```python
from build123d import *

# Parameters (mm, degrees)
SKETCH7_R           = 4.826
BOSS_EXTRUDE2_DEPTH = 9.652
SKETCH11_R          = 3.937
BOSS_EXTRUDE3_DEPTH = 7.874
RIB1_REACH          = 117.25
SKETCH16_WALL_W     = 293.372991472
SKETCH16_WALL_H     = 7.874
SKETCH17_R          = 9.525
SKETCH17_R_2        = 6.35
BOSS_EXTRUDE4_DEPTH = 14.986
SKETCH18_R          = 9.525
SKETCH18_R_2        = 6.35
BOSS_EXTRUDE5_DEPTH = 14.986


with BuildPart() as part:
    # Sketch7 → Boss-Extrude2 (new body)
    with BuildSketch(Plane(origin=(0, 0, 0), x_dir=(1, 0, 0), z_dir=(0, 1, 0))):
        with BuildLine():
            Line((-34.925, 38.1), (34.925, 38.1))
            ThreePointArc((34.925, 38.1), (43.905256121, 34.380256121), (47.625, 25.4))
            Line((47.625, 25.4), (47.625, -25.4))
            ThreePointArc((47.625, -25.4), (43.905256121, -34.380256121), (34.925, -38.1))
            Line((34.925, -38.1), (-34.925, -38.1))
            ThreePointArc((-34.925, -38.1), (-43.905256121, -34.380256121), (-47.625, -25.4))
            Line((-47.625, -25.4), (-47.625, 25.4))
            ThreePointArc((-47.625, 25.4), (-43.905256121, 34.380256121), (-34.925, 38.1))
        make_face()
        with Locations(Location((-34.925, 25.4, 0), (0, 0, 270))):
            Circle(SKETCH7_R, mode=Mode.SUBTRACT)
        with Locations(Location((34.925, 25.4, 0), (0, 0, 90))):
            Circle(SKETCH7_R, mode=Mode.SUBTRACT)
        with Locations(Location((34.925, -25.4, 0), (0, 0, 270))):
            Circle(SKETCH7_R, mode=Mode.SUBTRACT)
        with Locations(Location((-34.925, -25.4, 0), (0, 0, 90))):
            Circle(SKETCH7_R, mode=Mode.SUBTRACT)
    extrude(amount=-BOSS_EXTRUDE2_DEPTH)



with BuildPart() as body_2:
    # Sketch11 → Boss-Extrude3 (new body)
    with BuildSketch(Plane(origin=(0, 67.170783942, 38.781070191), x_dir=(0, 0.4999999999999983, -0.8660254037844396), z_dir=(0, -0.8660254037844396, -0.4999999999999983))):
        with BuildLine():
            Line((53.364432116, -23.876), (8.660432116, -23.876))
            ThreePointArc((8.660432116, -23.876), (3.092673321, -21.569758795), (0.786432116, -16.002))
            Line((0.786432116, -16.002), (0.786432116, 16.002))
            ThreePointArc((0.786432116, 16.002), (3.092673321, 21.569758795), (8.660432116, 23.876))
            Line((8.660432116, 23.876), (53.364432116, 23.876))
            ThreePointArc((53.364432116, 23.876), (58.932190911, 21.569758795), (61.238432116, 16.002))
            Line((61.238432116, 16.002), (61.238432116, -16.002))
            ThreePointArc((61.238432116, -16.002), (58.932190911, -21.569758795), (53.364432116, -23.876))
        make_face()
        with Locations((53.364432116, -16.002)):
            Circle(SKETCH11_R, mode=Mode.SUBTRACT)
        with Locations(Location((8.660432116, -16.002, 0), (0, 0, 180))):
            Circle(SKETCH11_R, mode=Mode.SUBTRACT)
        with Locations(Location((53.364432116, 16.002, 0), (0, 0, 180))):
            Circle(SKETCH11_R, mode=Mode.SUBTRACT)
        with Locations((8.660432116, 16.002)):
            Circle(SKETCH11_R, mode=Mode.SUBTRACT)
    extrude(amount=BOSS_EXTRUDE3_DEPTH)


with BuildPart() as part_1:
    add(part.part)

    add(body_2.part)  # Loft1 merges body 2
    # Sketch15 → Loft1 section 0
    with BuildSketch(Plane(origin=(0, 60.351699913, 34.844070191), x_dir=(1, 0, 0), z_dir=(0, -0.8660254037844397, -0.4999999999999983))):
        with BuildLine():
            Line((23.876, -36.297466608), (-23.876, -36.297466608))
            Line((-23.876, -36.297466608), (-23.876, -44.171466608))
            Line((-23.876, -44.171466608), (23.876, -44.171466608))
            Line((23.876, -44.171466608), (23.876, -36.297466608))
        make_face()
    # Sketch12 → Loft1 section 1
    with BuildSketch(Plane(origin=(0, 0, 0), x_dir=(1, 0, 0), z_dir=(0, 1, 0))):
        with BuildLine():
            Line((-47.625, 3.937), (47.625, 3.937))
            Line((47.625, 3.937), (47.625, -3.937))
            Line((47.625, -3.937), (-47.625, -3.937))
            Line((-47.625, -3.937), (-47.625, 3.937))
        make_face()
    loft()

    # Sketch16 wall → Rib1 (add, up to next)
    with BuildSketch(Plane(origin=(0, 30.372457985, 36.1315), x_dir=(0, 0.997906295589, -0.064676311144), z_dir=(0, 0.064676311144, 0.997906295589)), mode=Mode.PRIVATE) as rib1_sk1:
        Rectangle(SKETCH16_WALL_W, SKETCH16_WALL_H)
    rib1_tool1 = extrude(rib1_sk1.sketch, amount=-RIB1_REACH, mode=Mode.PRIVATE) - part_1.part
    add(rib1_tool1.solids().sort_by_distance((0, 30.372457985, 36.1315))[0])

    # Sketch17 → Boss-Extrude4 (add)
    with BuildSketch(Plane(origin=(0, 0.02645219, 3.936822263), x_dir=(1, 0, 0), z_dir=(0, 0.0067190212517474575, 0.9999774271219419))):
        with Locations((12.7, 35.025547213)):
            Circle(SKETCH17_R)
        with Locations(Location((12.7, 35.025547213, 0), (0, 0, 270))):
            Circle(SKETCH17_R_2, mode=Mode.SUBTRACT)
    extrude(amount=BOSS_EXTRUDE4_DEPTH)

    # Sketch18 → Boss-Extrude5 (add)
    with BuildSketch(Plane(origin=(0, 0.025189007, -3.936838834), x_dir=(-1, 0, 0), z_dir=(0, 0.006398151525432763, -0.9999795316190516))):
        with Locations(Location((-12.7, 34.808230427, 0), (0, 0, 90))):
            Circle(SKETCH18_R)
        with Locations(Location((-12.7, 34.808230427, 0), (0, 0, 90))):
            Circle(SKETCH18_R_2, mode=Mode.SUBTRACT)
    extrude(amount=BOSS_EXTRUDE5_DEPTH)


solid = part_1.part
```
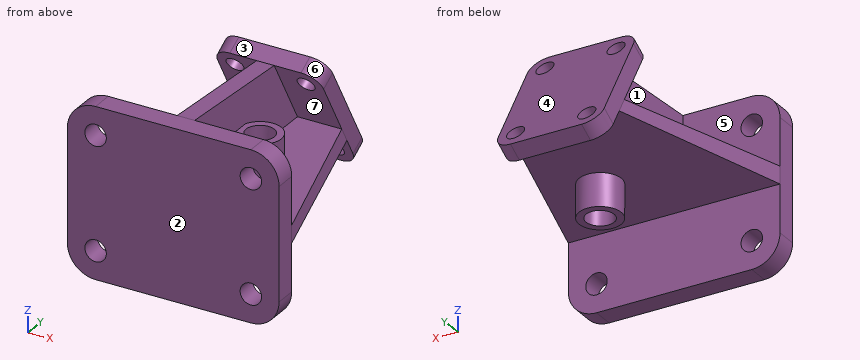
Geometry: final body of the model. Coordinates: model frame, mm. Face numbers are marked on the shaded views. A direction names the side the tool comes from. Round coordinates to 2 decimals unless told otherwise and drop trailing zeros. Write each loop counter-clockwise with the first axis right and the second up, starting at its lowest first coordinate (ties: lowest second). Pieces come first, ordered by that corner, then holes.
Item 1: Mould query, pull axis Y, two halves, no side actions, for the marked faces 1, 2, 3 and 4. Classes: +Y half, -Y half, draft (parallel to the pull), parting line (faces both ways), or undercut.
Item 2: Pin query (flat end, axial travel): P1, Ø7.5, axis at x = 34.925, z = -25.4, coming from the +Y side; P2, Ø23.5, axis at y = 82, z = 6, coming from the -X side; P3, Ø10, axis at x = -16.5, y = 59.5, coming from the -Z side; P4, Ø12.5, axis at x = -34.925, z = -25.4, coming from the +Y side. Return the tip coordinate at first contact, or that it passes through.
Item 3: Set-up query: the marked faces 5, 6 and 7. Return all of +Z, -Z, +X, -X, +Y, -Y with unobstructed straight access to the full face (end or side cutting, diameter ignored); none if empty.
Item 4: Section query A-A (x = -33.5). Give the number of separate pieces and of enclosed holes in the cut face, plus the area to 3 significant figures.
Item 5: Section query B-B (z = -33). Return loops of the section in (x, y), plus the area to 3 significant figures.
Item 6: Material intervals for L1, parallel to X at y = -4.5, z = 25.4 (3 decimals); L2, parallel to Z at x = 13, y = 67; L3, parallel to Z at x = 12, y = 26.5, sorted ascending.
Completed:
1. face 1: undercut
1. face 2: -Y half
1. face 3: undercut
1. face 4: +Y half
2. P1: passes through
2. P2: stops at x = -26.41
2. P3: stops at z = -3.59
2. P4: stops at y = 0
3. face 5: +Z, -X
3. face 6: +Z, +X
3. face 7: +X
4. separate pieces: 3
4. enclosed holes: 0
4. area: 919 mm2
5. outline: (-45.1, -9.65) - (45.1, -9.65) - (45.1, 0) - (-45.1, 0) - close
5. area: 871 mm2
6. L1: x = -47.625 to -39.751, -30.099 to 30.099, 39.751 to 47.625
6. L2: z = -3.51 to 3.49, 23.33 to 25.74, 31.62 to 37.77
6. L3: z = -18.75 to 18.75
